Geometry: final body of the model. Coordinates: model frame, mm. A direction names the side the tool comes from. Give positions to 0.01 mm unless a question says otherwise; leave off trailing zeros. Loops run counter-clockwise (first coordinate to the right, second up) from the corner with the lowest first, then second, coordinate; pieces in that order, holes last.
1. Access query for faces 5 (the face through (5.334, 5.273, 6.43)), 6 (the face through (-3.91, 3.87, 3.43)), 7 (the face through (0, -7.5, 6)). Directions: +Z, -Z, +X, -X, +Y, -Y. A direction counts if a zero-diameter tool reaches every point of the face in a straight line with its end or side. Return the directions, or none.
2. Section B-B, the plane y = 0. Output: boundary loops of the cut face in (x, z), then the cut area to 3 significant figures.
3. Draft query along X for faces 1 (the face through (3.91, -3.87, 3.43)), 2 (the face through (-5.334, -5.273, 6.43)), 3 (the face through (0.867, -3.905, 9.979)), 4 (the face through (0, -10, 0)). Return one class per face: +X half, -X half, draft (parallel to the pull), parting line (faces both ways), or undercut.
4. Material intervals for line 1 along Y through (x, z) = (0, 10.55); line 2 along Y through (x, z) = (-12, -0.45); line 3 along Z through (x, y) = (-13, -8.5), sorted ascending.
5. Section D-D, the plane z = 0.25. State how many separate pieces and enclosed holes the cut face has, then the cut area to 3 significant figures.
6. First-contact query: P1, Ø2, axis at y = 0, z = 5, coming from the -X side; P2, Ø10.5, axis at x = 0, y = 0, coming from the -Z side; P3, Ø4.5, axis at x = -1, z = 6, coming from the +Y side. Flat tips, straight axial feed; report the tip coordinate or a pass-through.
7. Section C-C, the plane x = 12. Output: boundary loops of the cut face in (y, z), then the cut area to 3 significant figures.
8. Section A-A, the plane x = 0. Output: boundary loops of the cut face in (y, z).
from build123d import *

# Parameters (mm, degrees)
F0_W         = 30
F0_H         = 3
F1_DEPTH     = 10
F3_DEPTH     = 10
F5_DEPTH     = 10
F7_D         = 8
F8_T1_DEPTH  = 10.517766953
F9_R         = 0.5
F10_T1_DEPTH = 10.517766953
F11_T1_DEPTH = 10.517766953
F12_T1_DEPTH = 10.517766953
F13_T1_DEPTH = 10.517766953
F14_T1_DEPTH = 10.517766953
F15_T1_DEPTH = 10.517766953
F17_D        = 3.3


# Not quite as in the source:
# - a fillet or chamfer that OpenCascade refuses, or shapes differently, is made with other operations: its cross-section is extruded or revolved along the edge and cut away or added
# - a feature names something its author has since deleted; it is built from what else it names


with BuildPart() as f1:
    # F0 (on Front) → F1 (new body, symmetric)
    with BuildSketch(Plane.XZ):
        Rectangle(F0_W, F0_H)
    extrude(amount=F1_DEPTH, both=True)

    # F2 (on face) → F3 (join)
    with BuildSketch(Plane.XY.offset(1.5)):
        Polygon((-3.1066017178, -7.5), (3.1066017178, -7.5), (7.5, -3.1066017178), (7.5, 3.1066017178), (3.1066017178, 7.5), (-3.1066017178, 7.5), (-7.5, 3.1066017178), (-7.5, -3.1066017178), align=None)
    extrude(amount=F3_DEPTH)

    # F4 (on face) → F5 (cut)
    with BuildSketch(Plane(origin=(0, 0, -1.5), x_dir=(1, 0, 0), z_dir=(0, 0, -1))):
        Polygon((-2.2781745931, -5.5), (2.2781745931, -5.5), (5.5, -2.2781745931), (5.5, 2.2781745931), (2.2781745931, 5.5), (-2.2781745931, 5.5), (-5.5, 2.2781745931), (-5.5, -2.2781745931), align=None)
    extrude(amount=-F5_DEPTH, mode=Mode.SUBTRACT)

    # F7 (through all)
    with Locations(Plane.XY.offset(11.5)):
        with Locations((0, 0)):
            Hole(F7_D / 2)

    # F8: fillet of radius 0.5 on 1 edges, made by hand

    # F8_s2 → F8_t1 (join)
    with BuildSketch(Plane.XY.offset(-1.5)):
        with BuildLine():
            add(Edge.make_bspline(
                [(2.4246212025, -5.3535533906), (2.2781745931, -5.5), (2.0710678119, -5.5)],
                knots=[0, 0, 0, 1, 1, 1], degree=2, weights=[1, 1, 1]))
            Line((2.0710678119, -5.5), (2.2781745931, -5.5))
            Line((2.2781745931, -5.5), (2.4246212025, -5.3535533906))
        make_face()
    extrude(amount=F8_T1_DEPTH)

    # F9
    f9_edges = [f1.edges().sort_by_distance(p)[0] for p in [
        (5.5, -2.278175, 3.5),
    ]]
    fillet(f9_edges, radius=F9_R)

    # F10: fillet of radius 0.5 on 1 edges, made by hand

    # F10_s2 → F10_t1 (join)
    with BuildSketch(Plane.XY.offset(-1.5)):
        with BuildLine():
            add(Edge.make_bspline(
                [(-2.0710678119, -5.5), (-2.2781745931, -5.5), (-2.4246212025, -5.3535533906)],
                knots=[0, 0, 0, 1, 1, 1], degree=2, weights=[1, 1, 1]))
            Line((-2.4246212025, -5.3535533906), (-2.2781745931, -5.5))
            Line((-2.2781745931, -5.5), (-2.0710678119, -5.5))
        make_face()
    extrude(amount=F10_T1_DEPTH)

    # F11: fillet of radius 0.5 on 1 edges, made by hand

    # F11_s2 → F11_t1 (join)
    with BuildSketch(Plane.XY.offset(-1.5)):
        with BuildLine():
            add(Edge.make_bspline(
                [(-5.3535533906, -2.4246212025), (-5.5, -2.2781745931), (-5.5, -2.0710678119)],
                knots=[0, 0, 0, 1, 1, 1], degree=2, weights=[1, 1, 1]))
            Line((-5.5, -2.0710678119), (-5.5, -2.2781745931))
            Line((-5.5, -2.2781745931), (-5.3535533906, -2.4246212025))
        make_face()
    extrude(amount=F11_T1_DEPTH)

    # F12: fillet of radius 0.5 on 1 edges, made by hand

    # F12_s2 → F12_t1 (join)
    with BuildSketch(Plane.XY.offset(-1.5)):
        with BuildLine():
            add(Edge.make_bspline(
                [(-5.3535533906, 2.4246212025), (-5.5, 2.2781745931), (-5.5, 2.0710678119)],
                knots=[0, 0, 0, 1, 1, 1], degree=2, weights=[1, 1, 1]))
            Line((-5.5, 2.0710678119), (-5.5, 2.2781745931))
            Line((-5.5, 2.2781745931), (-5.3535533906, 2.4246212025))
        make_face()
    extrude(amount=F12_T1_DEPTH)

    # F13: fillet of radius 0.5 on 1 edges, made by hand

    # F13_s2 → F13_t1 (join)
    with BuildSketch(Plane.XY.offset(-1.5)):
        with BuildLine():
            add(Edge.make_bspline(
                [(5.5, 2.0710678119), (5.5, 2.2781745931), (5.3535533906, 2.4246212025)],
                knots=[0, 0, 0, 1, 1, 1], degree=2, weights=[1, 1, 1]))
            Line((5.3535533906, 2.4246212025), (5.5, 2.2781745931))
            Line((5.5, 2.2781745931), (5.5, 2.0710678119))
        make_face()
    extrude(amount=F13_T1_DEPTH)

    # F14: fillet of radius 0.5 on 1 edges, made by hand

    # F14_s2 → F14_t1 (join)
    with BuildSketch(Plane.XY.offset(-1.5)):
        with BuildLine():
            add(Edge.make_bspline(
                [(2.4246212025, 5.3535533906), (2.2781745931, 5.5), (2.0710678119, 5.5)],
                knots=[0, 0, 0, 1, 1, 1], degree=2, weights=[1, 1, 1]))
            Line((2.0710678119, 5.5), (2.2781745931, 5.5))
            Line((2.2781745931, 5.5), (2.4246212025, 5.3535533906))
        make_face()
    extrude(amount=F14_T1_DEPTH)

    # F15: fillet of radius 0.5 on 1 edges, made by hand

    # F15_s2 → F15_t1 (join)
    with BuildSketch(Plane.XY.offset(-1.5)):
        with BuildLine():
            add(Edge.make_bspline(
                [(-2.0710678119, 5.5), (-2.2781745931, 5.5), (-2.4246212025, 5.3535533906)],
                knots=[0, 0, 0, 1, 1, 1], degree=2, weights=[1, 1, 1]))
            Line((-2.4246212025, 5.3535533906), (-2.2781745931, 5.5))
            Line((-2.2781745931, 5.5), (-2.0710678119, 5.5))
        make_face()
    extrude(amount=F15_T1_DEPTH)

    # F17 (through all)
    with Locations(Plane.XY.offset(1.5)):
        with Locations((-12, 0), (12, 0)):
            Hole(F17_D / 2)


solid = f1.part
Answers below:
1. face 5: +Z, +X, +Y
1. face 6: -Z
1. face 7: +Z, +X, -X, -Y
2. outline: (-15, -1.5) - (-13.65, -1.5) - (-13.65, 1.5) - (-15, 1.5) - close; (-10.35, -1.5) - (-5.5, -1.5) - (-5.5, 8.5) - (-4, 8.5) - (-4, 11.5) - (-7.5, 11.5) - (-7.5, 1.5) - (-10.35, 1.5) - close; (4, 8.5) - (5.5, 8.5) - (5.5, -1.5) - (10.35, -1.5) - (10.35, 1.5) - (7.5, 1.5) - (7.5, 11.5) - (4, 11.5) - close; (13.65, -1.5) - (15, -1.5) - (15, 1.5) - (13.65, 1.5) - close
2. area: 86.2 mm2
3. face 1: undercut
3. face 2: -X half
3. face 3: undercut
3. face 4: draft
4. line 1: y = -7.5 to -4, 4 to 7.5
4. line 2: y = -10 to -1.65, 1.65 to 10
4. line 3: z = -1.5 to 1.5
5. separate pieces: 1
5. enclosed holes: 3
5. area: 483 mm2
6. P1: stops at x = -7.5
6. P2: stops at z = 8.5
6. P3: stops at y = 7.5
7. outline: (-10, -1.5) - (-1.65, -1.5) - (-1.65, 1.5) - (-10, 1.5) - close; (1.65, -1.5) - (10, -1.5) - (10, 1.5) - (1.65, 1.5) - close
7. area: 50.1 mm2
8. outline: (-10, -1.5) - (-5.5, -1.5) - (-5.5, 8.5) - (-4, 8.5) - (-4, 11.5) - (-7.5, 11.5) - (-7.5, 1.5) - (-10, 1.5) - close; (4, 8.5) - (5.5, 8.5) - (5.5, -1.5) - (10, -1.5) - (10, 1.5) - (7.5, 1.5) - (7.5, 11.5) - (4, 11.5) - close
